Read the model definition and answer for the solid it produces. Units are mm, in the model's axes. Give positions to 0.01 mm unless a question says otherwise; leave off trailing zeros. Loops run counter-clockwise (first coordinate to the right, second up) from the corner with the lowest first, then second, coordinate; pieces in that order, holes last. Notation, with made-up numbers: (-21.5, 45.25) -> (8.5, 45.25) arc R12 cw to (8.5, 59.25) -> close; hole circle Ø11 at (69.25, -33). An arc over 180 degrees is marked (long way). Write each question's results on one line, items separated by ' | '. Start each with the question number.
Item 1: Determine the mould class of faces 1 (the flat face through (-1, 2, -50)), 2 (the cylindrical face through (-17.6, 1.97, 12.43)), 3 (the cylindrical face through (-49, 2, 48)) for opening direction Z: +Z half, -Z half, draft (parallel to the pull), parting line (faces both ways), or undercut.
Item 2: Section A-A on x = -16 is taken. Write down the section's boundary in (y, z).
Item 3: Section B-B on z = 12.5 is taken. Write down the section's boundary in (x, y).
Item 4: Find the intervals of material crossed by line 1 (X direction, y = 2.8, z = -45); line 2 (X direction, y = 2.7, z = 12.5), in increasing order.
Item 5: This flat-tipped pin is pushed along its axis until it touches: P1, Ø1, axis at x = 28.5, z = 33.5, coming from the -Y side. Where does it stop, or does it pass through?
```python
from build123d import *

# Parameters (mm, degrees)
SKETCH1_W           = 100
SKETCH1_H           = 100
SKETCH1_R           = 1.6
BOSS_EXTRUDE1_DEPTH = 4
FILLET1_R           = 5


with BuildPart() as part:
    # Sketch1 → Boss-Extrude1 (new body)
    with BuildSketch(Plane(origin=(0, 0, 0), x_dir=(1, 0, 0), z_dir=(0, 1, 0))):
        Rectangle(SKETCH1_W, SKETCH1_H)
        with Locations((-45, 45)):
            Circle(SKETCH1_R, mode=Mode.SUBTRACT)
        with Locations((45, 45)):
            Circle(SKETCH1_R, mode=Mode.SUBTRACT)
        with Locations((45, -45)):
            Circle(SKETCH1_R, mode=Mode.SUBTRACT)
        with Locations((-45, -45)):
            Circle(SKETCH1_R, mode=Mode.SUBTRACT)
        with Locations((16, -12.5)):
            Circle(SKETCH1_R, mode=Mode.SUBTRACT)
        with Locations((-16, -12.5)):
            Circle(SKETCH1_R, mode=Mode.SUBTRACT)
    extrude(amount=BOSS_EXTRUDE1_DEPTH)

    # Fillet1
    fillet1_edges = [part.edges().sort_by_distance(p)[0] for p in [
        (-50, 2, -50),
        (50, 2, -50),
        (50, 2, 50),
        (-50, 2, 50),
    ]]
    fillet(fillet1_edges, radius=FILLET1_R)


solid = part.part
```
Findings:
1) face 1: -Z half | face 2: undercut | face 3: +Z half
2) outline: (0, -50) -> (4, -50) -> (4, 10.9) -> (0, 10.9) -> close; (0, 14.1) -> (4, 14.1) -> (4, 50) -> (0, 50) -> close
3) outline: (-50, 0) -> (-17.6, 0) -> (-17.6, 4) -> (-50, 4) -> close; (-14.4, 0) -> (14.4, 0) -> (14.4, 4) -> (-14.4, 4) -> close; (17.6, 0) -> (50, 0) -> (50, 4) -> (17.6, 4) -> close
4) line 1: -50 to -46.6, -43.4 to 43.4, 46.6 to 50 | line 2: -50 to -17.6, -14.4 to 14.4, 17.6 to 50
5) P1: y = 0
